Could you check a few things on this drawing? It's one solid part, dimensions in mm from its lowest x, y, z. A direction names the side the tool comes from. Coordinates: 2 decimals unless noted, no trailing zeros. Order: outer loops, then holes, each group sorted by start corner. A loop starts at its lowest first (then second) coordinate and runs counter-clockwise, first axis right, second up. Notation, with made-up numbers: (86, 13) -> (116, 13) arc R17 cw to (116, 24) -> close; hole circle Ø1 at (4.5, 15). An arc over 180 degrees is marked (long way). Use a Markdown table: item, result. Add a question column.
1. We'd pull the mould along Z, two halves only. Please class the marked faces 1, 2 and 3: pulls with the +Z half, pulls with the -Z half, needs draft (parallel to the pull), parting line crosses it, or undercut.
2. Suppose I cut it at A-A, the plane x = 9.5. List the corners of the cut face in (y, z) for me.
3. For pin 1 Ø1 at (x, z) = (6, 10.5) entering from -Y; pin 2 Ø1 at (x, y) = (12.5, 11) entering from -Z; pin 3 Ø2 at (x, z) = (7.5, 11) entering from +Y, each with a flat end and sliding along its axis, tell me the tip position at first contact or that it passes through.
4. For the marked faces 4, 5 and 6, which set-ups out of +Z, -Z, +X, -X, +Y, -Y let a thin tool reach every point of the face, with its end or its side?
5. Suppose I cut it at B-B, the plane z = 6.5. List the corners of the cut face in (x, y) for me.
6. Suppose I cut it at C-C, the plane y = 11. List the corners of the cut face in (x, z) for me.
7. Suppose I cut it at D-D, the plane x = 1.5. List the corners of the cut face in (y, z) for me.
8. If I drill on line 1 along Z through (x, y) = (9.5, 1.5); line 2 along Z through (x, y) = (11.5, 1.5); line 3 along X through (y, z) = (9.75, 14.25), over which ranges is the centre line in solid material (lowest first)? Write a range as from..to.
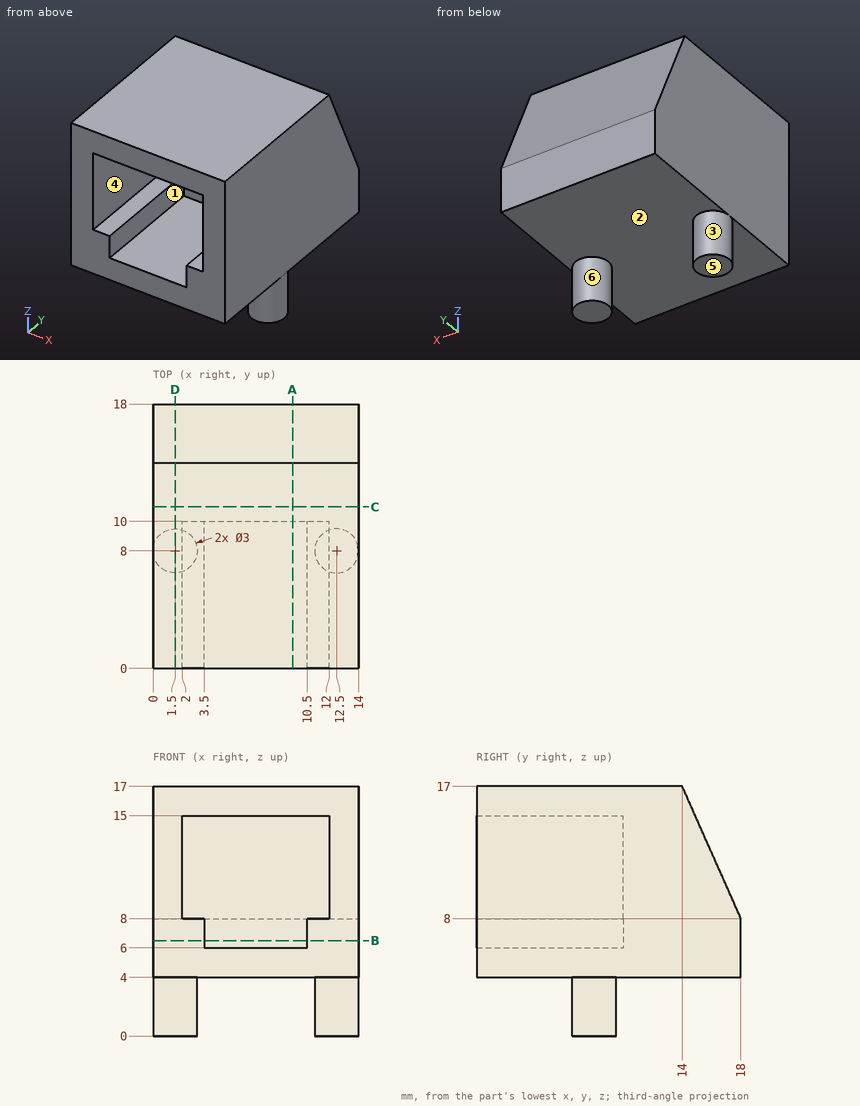
Worked out:
| question | item | result |
|---|---|---|
| 1 | face 1 | undercut |
| 1 | face 2 | pulls with the -Z half |
| 1 | face 3 | needs draft |
| 2 | outline | (0, 4) -> (18, 4) -> (18, 8) -> (14, 17) -> (0, 17) -> (0, 15) -> (10, 15) -> (10, 6) -> (0, 6) -> close |
| 3 | pin 1 | stops at y = 10 |
| 3 | pin 2 | stops at z = 4 |
| 3 | pin 3 | stops at y = 17.11 |
| 4 | face 4 | -Y |
| 4 | face 5 | -Z, +X, -X, +Y, -Y |
| 4 | face 6 | -Z |
| 5 | outline | (0, 0) -> (3.5, 0) -> (3.5, 10) -> (10.5, 10) -> (10.5, 0) -> (14, 0) -> (14, 18) -> (0, 18) -> close |
| 6 | outline | (0, 4) -> (14, 4) -> (14, 17) -> (0, 17) -> close |
| 7 | outline | (0, 4) -> (6.5, 4) -> (6.5, 0) -> (9.5, 0) -> (9.5, 4) -> (18, 4) -> (18, 8) -> (14, 17) -> (0, 17) -> close |
| 8 | line 1 | z = 4..6, 15..17 |
| 8 | line 2 | z = 4..8, 15..17 |
| 8 | line 3 | x = 0..2, 12..14 |
